Input: part model. Units: mm. Frame: model coordinates. A direction names the side the tool comes from. Coordinates: 2 decimals unless noted, no trailing zeros. Write each loop counter-clockwise with the first axis right and the second up, starting at its lowest first coordinate (ties: lowest second). Pieces come first, ordered by that corner, then holes. Notation, with made-up numbers: (-12, 1) -> (20, 1) arc R25 ccw to (20, 19) -> close; hole circle Ø5 at (-27.5, 11.25). An arc over 180 degrees is marked (long way). Use one line per item in the form item = value. Start each with the question number.
(1) Set-up query: faces 1 (the face through (-1, 18, -60)), 2 (the face through (-1, 14, -49.932)). Return all of +Z, -Z, +X, -X, +Y, -Y with unobstructed straight access to the full face (end or side cutting, diameter ignored); none if empty.
(2) Ray query, line 1 along Z through (x, y) = (0, 3.5); line 2 along Y through (x, z) = (-64, -26). Return the intervals inside material, ascending.
(3) Cut plane D-D on x = 43. Return the cut outline in (y, z), plus the area to 3 significant figures.
(4) First-contact query: pin 1 (10 mm diameter, centred on x = 34, z = -5.5, fed in from +Y); pin 2 (4.5 mm diameter, centred on x = 4, y = 12, fed in from -Z); pin 3 (2 mm diameter, centred on x = -27, z = -2, fed in from -Y); pin 4 (4 mm diameter, centred on y = 9.5, z = -43, fed in from -X). Flat tips, straight axial feed; report the tip coordinate or a pass-through.
(5) Cut plane B-B on z = 0. Return the cut outline in (x, y), plus the area to 3 significant figures.
(6) Pull-direction query (Z, two-part tool) for faces 3 (the face through (-9.894, 6.874, -75.353)), 4 (the face through (-3, 5, 0)), 5 (the face through (-1, 0, 16)), 6 (the face through (1, 14, 49.932)); classes: released by +Z, released by -Z, zero draft, split by the parting line, or undercut.
(7) Cut plane C-C on y = 14. Return the cut outline in (x, z).
(8) Cut plane A-A on x = 0. Return the cut outline in (y, z).
```python
from build123d import *

# Parameters (mm, degrees)
SKETCH1_R           = 76
BOSS_EXTRUDE1_DEPTH = 18
CUT_EXTRUDE4_DEPTH  = 8.89
SKETCH5_R           = 3
CUT_EXTRUDE5_DEPTH  = 20


with BuildPart() as part:
    # Sketch1 → Boss-Extrude1 (new body)
    with BuildSketch(Plane(origin=(0, 0, 0), x_dir=(1, 0, 0), z_dir=(0, 1, 0))):
        Circle(SKETCH1_R)
    extrude(amount=BOSS_EXTRUDE1_DEPTH)

    # Sketch2 → Cut-Extrude4 (cut)
    with BuildSketch(Plane(origin=(0, 18, 0), x_dir=(1, 0, 0), z_dir=(0, 1, 0))):
        with BuildLine():
            Line((-58.007955522, 49.931796385), (58.007955522, 49.931796385))
            ThreePointArc((58.007955522, 49.931796385), (107.939751907, 0), (58.007955522, -49.931796385))
            Line((58.007955522, -49.931796385), (-58.007955522, -49.931796385))
            ThreePointArc((-58.007955522, -49.931796385), (-107.939751907, 0), (-58.007955522, 49.931796385))
        make_face()
    extrude(amount=-CUT_EXTRUDE4_DEPTH, mode=Mode.SUBTRACT)

    # Sketch5 → Cut-Extrude5 (cut)
    with BuildSketch(Plane(origin=(0, 9.11, 0), x_dir=(1, 0, 0), z_dir=(0, 1, 0))):
        Circle(SKETCH5_R)
    extrude(amount=-CUT_EXTRUDE5_DEPTH, mode=Mode.SUBTRACT)


solid = part.part
```
Values:
q1.face_1 = +Z, -Z, +X, -X, +Y
q1.face_2 = +X, -X, +Y
q2.line_1 = -76 to -3, 3 to 76
q2.line_2 = 0 to 9.11
q3.outline = (0, -62.67) -> (18, -62.67) -> (18, -49.93) -> (9.11, -49.93) -> (9.11, 49.93) -> (18, 49.93) -> (18, 62.67) -> (0, 62.67) -> close
q3.area = 1,370 mm2
q4.pin_1 = 9.11
q4.pin_2 = -75.98
q4.pin_3 = 0
q4.pin_4 = -63.97
q5.outline = (-76, 0) -> (-3, 0) -> (-3, 9.11) -> (-76, 9.11) -> close; (3, 0) -> (76, 0) -> (76, 9.11) -> (3, 9.11) -> close
q5.area = 1,330 mm2
q6.face_3 = split by the parting line
q6.face_4 = undercut
q6.face_5 = zero draft
q6.face_6 = undercut
q7.outline = (-57.3, -49.93) arc R76 ccw to (57.3, -49.93) -> close; (-57.3, 49.93) -> (57.3, 49.93) arc R76 ccw to start
q8.outline = (0, -76) -> (18, -76) -> (18, -49.93) -> (9.11, -49.93) -> (9.11, -3) -> (0, -3) -> close; (0, 3) -> (9.11, 3) -> (9.11, 49.93) -> (18, 49.93) -> (18, 76) -> (0, 76) -> close
